Autodesk Inventor part; units mm, degrees
ref_plane "YZ Plane" through (0, 0, 0) normal (1, 0, 0) x (0, 1, 0)
ref_plane "XZ Plane" through (0, 0, 0) normal (0, 1, 0) x (-1, 0, 0)
ref_plane "XY Plane" through (0, 0, 0) normal (0, 0, 1) x (1, 0, 0)
sketch "Sketch1" plane through (0, 0, 0) normal (0, 1, 0) x (-1, 0, 0)
  line L0 (0, 0) -> (1219.2, 0)
  line L1 (1219.2, 0) -> (1219.2, 1371.6)
  line L2 (1219.2, 1371.6) -> (0, 1371.6)
  line L3 (0, 1371.6) -> (0, 0)
  dimension "d0" = 1219.2
  dimension "d1" = 1371.6
extrude "Plate1" add sketch "Sketch1" along normal blind 5.3975
sketch "Sketch2" plane through (0, 0, 1366.2025) normal (0, 0, 1) x (1, 0, 0)
  line L0 (-1219.2, 0) -> (0, 0)
  line L1 (0, 0) -> (0, 25.4)
  line L2 (0, 25.4) -> (-1219.2, 25.4)
  line L3 (-1219.2, 25.4) -> (-1219.2, 0)
edge flange "Flange1" height 25.4 angle 90 thickness 5.3975 bend radius 5.3975 thickness toward (0, 0, 1) relief tear relief width 5.3975 relief depth 2.6987 edges at (-609.6, 5.3975, 1371.6) wall of the first edge with corners at (-1219.2, 0, 1366.2025) (0, 0, 1366.2025) (0, 25.4, 1366.2025) (-1219.2, 25.4, 1366.2025)
bend "Bend1"
corner "Corner1"
sketch "Sketch3" plane through (0, 20.0025, 1371.6) normal (0, 1, 0) x (-1, 0, 0)
  line L0 (1219.2, 0) -> (0, 0)
  line L1 (0, 0) -> (0, -25.4)
  line L2 (0, -25.4) -> (1219.2, -25.4)
  line L3 (1219.2, -25.4) -> (1219.2, 0)
edge flange "Flange2" height 25.4 angle 90 thickness 5.3975 bend radius 5.3975 thickness toward (0, 1, 0) relief tear relief width 5.3975 relief depth 2.6987 edges at (-609.6, 25.4, 1366.2025) wall of the first edge with corners at (-1219.2, 20.0025, 1371.6) (0, 20.0025, 1371.6) (0, 20.0025, 1346.2) (-1219.2, 20.0025, 1346.2)
bend "Bend2"
corner "Corner2"
equation "\"d3\" = BendReliefWidth"
equation "\"d4\" = BendReliefDepth"
equation "\"d5\" = MinimumRemnant"
equation "\"d6\" = BendRadius"
equation "\"d9\" = BendRadius"
equation "\"d10\" = CornerReliefSize"
equation "\"d11\" = GapSize"
equation "\"d12\" = JacobiRadiusSize"
equation "\"d13\" = BendReliefWidth"
equation "\"d14\" = BendReliefDepth"
equation "\"d15\" = MinimumRemnant"
equation "\"d16\" = BendRadius"
equation "\"d19\" = BendRadius"
equation "\"d20\" = CornerReliefSize"
equation "\"d21\" = GapSize"
equation "\"d22\" = JacobiRadiusSize"
equation "\"BendRadius\" = Thickness"
equation "\"BendReliefWidth\" = Thickness"
equation "\"BendReliefDepth\" = 0.5 * Thickness"
equation "\"CornerReliefSize\" = 4 * Thickness"
equation "\"MinimumRemnant\" = 2 * Thickness"
equation "\"TransitionRadius\" = BendRadius"
equation "\"JacobiRadiusSize\" = BendRadius"
equation "\"GapSize\" = Thickness"
equation "\"d2\" = BendRadius"
properties part number "wall-side" material "Polycarbonate, Clear"
Geometry check sheet. Reference: the model listing, model coordinates, mm. Round coordinates to 2 decimals unless told otherwise and drop trailing zeros. Loops run counter-clockwise (first coordinate to the right, second up) from the corner with the lowest first, then second, coordinate; pieces in that order, holes last. Notation, with made-up numbers: (26, 52.25) - (33, 52.25) arc R28 cw to (33, 82.25) - close; hole circle Ø10 at (55, -9). An arc over 180 degrees is marked (long way). Write item = value, one per line. Start each with the question number.
1. Section check B-B on z = 742. Enter the section's corners in (x, y).
2. Section check A-A on x = -523. Enter the section's corners in (y, z) (1 decimal).
3. Depth check by flat-ended pin: pin 1 (8 mm diameter, centred on x = -891.5, z = 919, fed in from +Y); pin 2 (4.5 mm diameter, centred on x = -810.5, y = 23, fed in from -Z); pin 3 (10 mm diameter, centred on y = 13, z = 749, fed in from +X); pin 4 (3 mm diameter, centred on x = -325.5, y = 13, fed in from -Z). Enter the tip coordinate at first touch or a pass-through.
4. Thickness scan on line 1 (Z direction, x = -329, y = 23.75); line 2 (Y direction, x = -144, z = 69.5); line 3 (Z direction, x = -519, y = 10.75). Record the ranges inside material, lowest first.
Working result:
q1.outline = (-1219.2, 0) - (0, 0) - (0, 5.4) - (-1219.2, 5.4) - close
q2.outline = (0, 0) - (5.4, 0) - (5.4, 1360.8) arc R5.4 cw to (10.8, 1366.2) - (14.6, 1366.2) arc R5.4 cw to (20, 1360.8) - (20, 1346.2) - (25.4, 1346.2) - (25.4, 1360.8) arc R10.8 ccw to (14.6, 1371.6) - (10.8, 1371.6) arc R10.8 ccw to (0, 1360.8) - close
q3.pin_1 = 5.4
q3.pin_2 = 1346.2
q3.pin_3 = through
q3.pin_4 = 1366.2
q4.line_1 = 1346.2 to 1366.54
q4.line_2 = 0 to 5.4
q4.line_3 = 1366.2 to 1371.6
